from build123d import *

# Parameters (mm, degrees)
SKETCH2_R           = 1.6
SKETCH2_R_2         = 2.15265
BOSS_EXTRUDE1_DEPTH = 2.54


with BuildPart() as part:
    # Sketch2 → Boss-Extrude1 (new body)
    with BuildSketch(Plane(origin=(0, 0, 0), x_dir=(1, 0, 0), z_dir=(0, 1, 0))):
        with BuildLine():
            Line((-55.5625, -36.5125), (55.5625, -36.5125))
            ThreePointArc((55.5625, -36.5125), (57.80756403, -35.58256403), (58.7375, -33.3375))
            Line((58.7375, -33.3375), (58.7375, 33.3375))
            ThreePointArc((58.7375, 33.3375), (57.80756403, 35.58256403), (55.5625, 36.5125))
            Line((55.5625, 36.5125), (-55.5625, 36.5125))
            ThreePointArc((-55.5625, 36.5125), (-57.80756403, 35.58256403), (-58.7375, 33.3375))
            Line((-58.7375, 33.3375), (-58.7375, -33.3375))
            ThreePointArc((-58.7375, -33.3375), (-57.80756403, -35.58256403), (-55.5625, -36.5125))
        make_face()
        with Locations(Location((9.5, 0, 0), (0, 0, 270))):
            Circle(SKETCH2_R, mode=Mode.SUBTRACT)
        with Locations(Location((31.5, 0, 0), (0, 0, 270))):
            Circle(SKETCH2_R, mode=Mode.SUBTRACT)
        with Locations(Location((47.625, 25.4, 0), (0, 0, 90))):
            Circle(SKETCH2_R_2, mode=Mode.SUBTRACT)
        with Locations(Location((47.625, -25.4, 0), (0, 0, 270))):
            Circle(SKETCH2_R_2, mode=Mode.SUBTRACT)
        with Locations(Location((-47.625, 25.4, 0), (0, 0, 270))):
            Circle(SKETCH2_R_2, mode=Mode.SUBTRACT)
        with Locations(Location((-47.625, -25.4, 0), (0, 0, 90))):
            Circle(SKETCH2_R_2, mode=Mode.SUBTRACT)
        with BuildLine():
            Line((14.5, -6.85), (26.5, -6.85))
            ThreePointArc((26.5, -6.85), (27.454594155, -6.454594155), (27.85, -5.5))
            Line((27.85, -5.5), (27.85, 5.5))
            ThreePointArc((27.85, 5.5), (27.454594155, 6.454594155), (26.5, 6.85))
            Line((26.5, 6.85), (14.5, 6.85))
            ThreePointArc((14.5, 6.85), (13.545405845, 6.454594155), (13.15, 5.5))
            Line((13.15, 5.5), (13.15, -5.5))
            ThreePointArc((13.15, -5.5), (13.545405845, -6.454594155), (14.5, -6.85))
        make_face(mode=Mode.SUBTRACT)
        with BuildLine():
            Line((-7.9, 15.95), (-31.1, 15.95))
            ThreePointArc((-31.1, 15.95), (-32.514213562, 15.364213562), (-33.1, 13.95))
            Line((-33.1, 13.95), (-33.1, -13.95))
            ThreePointArc((-33.1, -13.95), (-32.514213562, -15.364213562), (-31.1, -15.95))
            Line((-31.1, -15.95), (-7.9, -15.95))
            ThreePointArc((-7.9, -15.95), (-6.485786438, -15.364213562), (-5.9, -13.95))
            Line((-5.9, -13.95), (-5.9, 13.95))
            ThreePointArc((-5.9, 13.95), (-6.485786438, 15.364213562), (-7.9, 15.95))
        make_face(mode=Mode.SUBTRACT)
    extrude(amount=BOSS_EXTRUDE1_DEPTH)


solid = part.part
Here's how the part is built. I have some questions about the finished solid (model axes, mm). A direction names the side the tool comes from. Give positions to 0.01 mm unless a question says otherwise; leave off trailing zeros. Loops run counter-clockwise (first coordinate to the right, second up) from the corner with the lowest first, then second, coordinate; pieces in that order, holes last. Notation, with made-up numbers: (-24.75, 68) -> (-4.75, 68) arc R16 cw to (-4.75, 93) -> close; hole circle Ø4 at (-24, -40). An arc over 180 degrees is marked (long way). One line per item, written item: value.
Q1. Suppose I cut it at C-C on x = -14. Please give me the cut outline in (y, z).
Answers follow:
outline: (0, -36.51) -> (2.54, -36.51) -> (2.54, -15.95) -> (0, -15.95) -> close; (0, 15.95) -> (2.54, 15.95) -> (2.54, 36.51) -> (0, 36.51) -> close
Q2. Suppose I cut it at A-A on z = 25.4. Please give me the cut outline in (x, y), then the cut area to 3 significant figures.
Answers follow:
outline: (-58.74, 0) -> (-49.78, 0) -> (-49.78, 2.54) -> (-58.74, 2.54) -> close; (-45.47, 0) -> (45.47, 0) -> (45.47, 2.54) -> (-45.47, 2.54) -> close; (49.78, 0) -> (58.74, 0) -> (58.74, 2.54) -> (49.78, 2.54) -> close
area: 277 mm^2
Q3. If I drill on line 1 along X through (y, z) = (1, -25.4); line 2 along X through (y, z) = (0.9, -3); line 3 along X through (y, z) = (0.65, 0), over which ranges is the centre line in solid material (lowest first)?
Answers follow:
line 1: -58.74 to -49.78, -45.47 to 45.47, 49.78 to 58.74
line 2: -58.74 to -33.1, -5.9 to 13.15, 27.85 to 58.74
line 3: -58.74 to -33.1, -5.9 to 7.9, 11.1 to 13.15, 27.85 to 29.9, 33.1 to 58.74
Q4. Suppose I cut it at D-D on y = 0.75. State how many separate pieces and enclosed holes the cut face has, then the cut area to 3 significant figures.
Answers follow:
separate pieces: 1
enclosed holes: 8
area: 7,430 mm^2
Q5. Suppose I cut it at B-B on x = 23. Please give me the cut outline in (y, z), then the cut area to 3 significant figures.
Answers follow:
outline: (0, -36.51) -> (2.54, -36.51) -> (2.54, -6.85) -> (0, -6.85) -> close; (0, 6.85) -> (2.54, 6.85) -> (2.54, 36.51) -> (0, 36.51) -> close
area: 151 mm^2
Q6. We'd pull the mould along X, two halves only. Please class faces 1 (the face through (-20, 1, 15.95)), 2 (the face through (-57.78, 1.25, -35.61)), 3 (the face through (57.83, 1.25, -35.56)), 4 (the face through (-1, 1, 36.512)): pulls with the +X half, pulls with the -X half, needs draft (parallel to the pull), parting line crosses it, or undercut.
Answers follow:
face 1: undercut
face 2: pulls with the -X half
face 3: pulls with the +X half
face 4: needs draft
Q7. On a 3-axis mill with a long thin cutter (end or side, diameter ignored), from which of +Z, -Z, +X, -X, +Y, -Y can I reach the whole of each face in a straight line? I mean faces 5 (the face through (58.738, 1, 0)), 6 (the face through (13.15, 1, 0)). Say none if no direction works.
Answers follow:
face 5: +Z, -Z, +X, +Y, -Y
face 6: +Y, -Y
